For this review, use the dimensioned drawing (mm, ordinates from the lowest corner) and the shaded views. Give positions to 0.01 mm unless a question says otherwise; leave off trailing zeros. Order: outer loops, then holes, each group sorted by start corner. A loop starts at its lowest first (then second) coordinate and runs counter-clockwise, first axis right, second up.
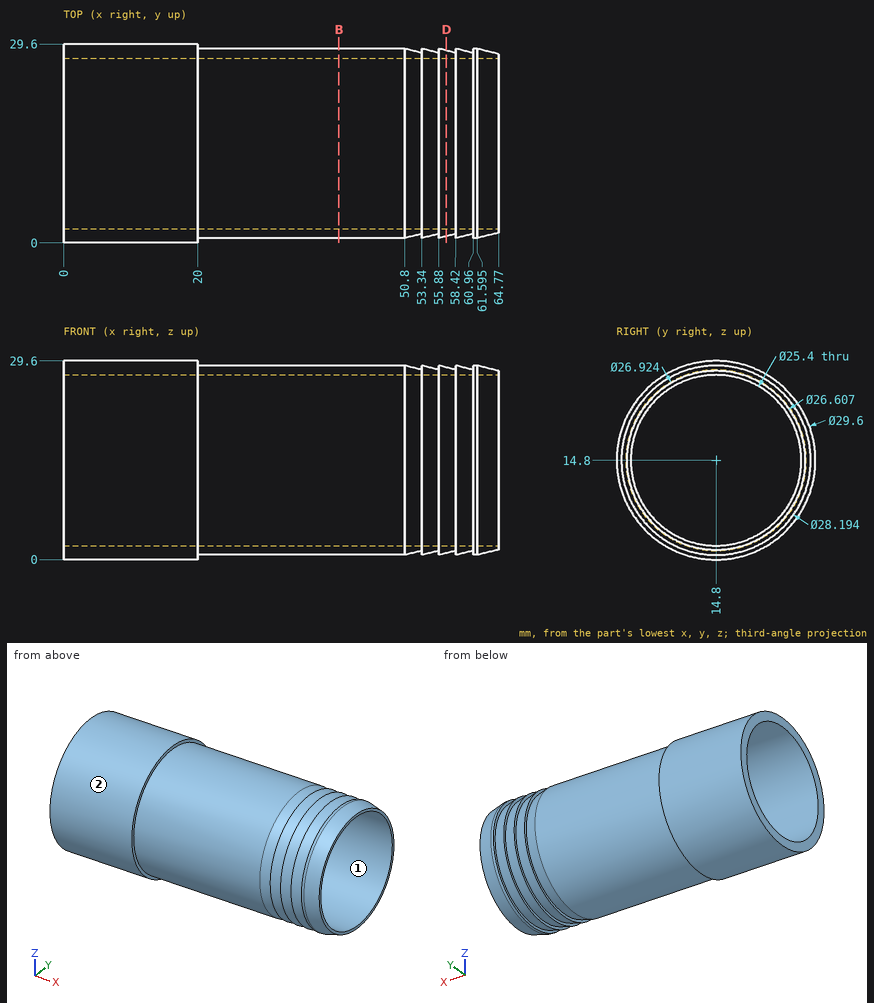
1. Take a section at B-B (x = 41). State the section outline as (y, z) points (1 decimal).
Recorded:
outline: circle Ø28.2 at (14.8, 14.8); hole circle Ø25.4 at (14.8, 14.8)
2. For pin 1 (14 mm diameter, centred on y = 18, z = 18.5, fed in from -X); pin 2 (12 mm diameter, centred on x = 55.5, z = 20.5, fed in from -Y); pin 3 (4 mm diameter, centred on x = 53.5, z = 26.5, fed in from +Y) (1 decimal), all flat-tipped, find the tip position at first contact; note any pin that passes through.
Recorded:
pin 1: passes through
pin 2: stops at y = 0.7
pin 3: stops at y = 25
3. Take a section at D-D (x = 57). State the section outline as (y, z) points (1 decimal).
Recorded:
outline: circle Ø27.6 at (14.8, 14.8); hole circle Ø25.4 at (14.8, 14.8)
4. Draft analysis for pull direction Y (two halves, no side actions). For the marked faces 1 and 2, state which applies: pulls with the +Y half, pulls with the -Y half, needs draft (parallel to the pull), parting line crosses it, or undercut.
Recorded:
face 1: undercut
face 2: parting line crosses it
5. For line 1 along Y through (x, z) = (24, 14.8); line 2 along Y through (x, z) = (13.5, 15.25); line 3 along Z through (x, y) = (8.5, 17.25) (1 decimal), list the stretches that pass through material, from the lowest coordinate up.
Recorded:
line 1: y = 0.7 to 2.1, 27.5 to 28.9
line 2: y = 0.01 to 2.11, 27.49 to 29.59
line 3: z = 0.2 to 2.3, 27.3 to 29.4
